from build123d import *

# Parameters (mm, degrees)
SKETCH1_R            = 1
BOSS_EXTRUDE1_DEPTH  = 6
SKETCH2_R            = 2.6
CUT_EXTRUDE1_DEPTH   = 6
SKETCH3_W            = 7.6
SKETCH3_H            = 13
BOSS_EXTRUDE2_DEPTH  = 6
BOSS_EXTRUDE5_START  = -5
SKETCH6_W            = 3
SKETCH6_H            = 2
BOSS_EXTRUDE5_DEPTH  = 13
BOSS_EXTRUDE6_START  = -6
SKETCH10_R           = 4
SKETCH10_R_2         = 2.6
BOSS_EXTRUDE6_DEPTH  = 1.5
BOSS_EXTRUDE7_START  = -6
SKETCH12_R           = 2.6
SKETCH12_R_2         = 2.4
BOSS_EXTRUDE7_DEPTH  = 2
CUT_EXTRUDE2_DEPTH   = 7
SKETCH14_W           = 3
SKETCH14_H           = 6
CUT_EXTRUDE3_DEPTH   = 2
SKETCH15_W           = 0.2
SKETCH15_H           = 13
CUT_EXTRUDE5_DEPTH   = 7.5
SKETCH16_W           = 3
SKETCH16_H           = 3
CUT_EXTRUDE6_DEPTH   = 3
SKETCH17_W           = 2.8
SKETCH17_H           = 2.8
BOSS_EXTRUDE9_DEPTH  = 3
BOSS_EXTRUDE10_START = 24.4
SKETCH17_2_W         = 2.8
SKETCH17_2_H         = 2.8
BOSS_EXTRUDE10_DEPTH = 3
SKETCH18_W           = 5.7
SKETCH18_H           = 13
SKETCH18_W_2         = 13.3
CUT_EXTRUDE7_DEPTH   = 9
SKETCH19_W           = 3
SKETCH19_H           = 3
CUT_EXTRUDE8_DEPTH   = 3
CUT_EXTRUDE10_START  = -24
SKETCH19_3_W         = 3
SKETCH19_3_H         = 3
CUT_EXTRUDE10_DEPTH  = 3


with BuildPart() as part:
    # Sketch1 → Boss-Extrude1 (new body)
    with BuildSketch(Plane.XY):
        with BuildLine():
            ThreePointArc((3.75, -5), (4.47902769, -4.358991965), (5.1, -3.61282438))
            Line((5.1, -3.61282438), (5.1, 3.61282438))
            ThreePointArc((5.1, 3.61282438), (0, 6.25), (-5.1, 3.61282438))
            Line((-5.1, 3.61282438), (-5.1, -3.61282438))
            ThreePointArc((-5.1, -3.61282438), (-4.47902769, -4.358991965), (-3.75, -5))
            Line((-3.75, -5), (-14.7, -5))
            Line((-14.7, -5), (-14.7, 8))
            Line((-14.7, 8), (14.7, 8))
            Line((14.7, 8), (14.7, -5))
            Line((14.7, -5), (3.75, -5))
        make_face()
        with Locations((11.5, 0)):
            Circle(SKETCH1_R, mode=Mode.SUBTRACT)
        with Locations((-11.5, 0)):
            Circle(SKETCH1_R, mode=Mode.SUBTRACT)
    extrude(amount=BOSS_EXTRUDE1_DEPTH)

    # Sketch2 → Cut-Extrude1 (cut)
    with BuildSketch(Plane.XY):
        with Locations((-11.5, 0)):
            Circle(SKETCH2_R)
        with Locations((11.5, 0)):
            Circle(SKETCH2_R)
    extrude(amount=CUT_EXTRUDE1_DEPTH, mode=Mode.SUBTRACT)

    # Sketch3 → Boss-Extrude2 (add)
    with BuildSketch(Plane.XY):
        with Locations((-18.5, 1.5)):
            Rectangle(SKETCH3_W, SKETCH3_H)
    extrude(amount=BOSS_EXTRUDE2_DEPTH)

    # Sketch6 → Boss-Extrude5 (add)
    with BuildSketch(Plane(origin=(0, 0, 0), x_dir=(1, 0, 0), z_dir=(0, 1, 0)).offset(BOSS_EXTRUDE5_START)):
        with Locations((-23.8, -3)):
            Rectangle(SKETCH6_W, SKETCH6_H)
        with Locations((16.2, -3)):
            Rectangle(SKETCH6_W, SKETCH6_H)
    extrude(amount=BOSS_EXTRUDE5_DEPTH)

    # Sketch10 → Boss-Extrude6 (add)
    with BuildSketch(Plane.XY.offset(6).offset(BOSS_EXTRUDE6_START)):
        with Locations((-11.5, 0)):
            Circle(SKETCH10_R)
        with Locations((-11.5, 0)):
            Circle(SKETCH10_R_2, mode=Mode.SUBTRACT)
        with BuildLine():
            Line((14.7, 2.4), (14.7, -2.4))
            ThreePointArc((14.7, -2.4), (7.5, 0), (14.7, 2.4))
        make_face()
        with Locations((11.5, 0)):
            Circle(SKETCH10_R_2, mode=Mode.SUBTRACT)
    extrude(amount=-BOSS_EXTRUDE6_DEPTH)

    # Sketch12 → Boss-Extrude7 (add)
    with BuildSketch(Plane(origin=(0, 0, 0), x_dir=(-1, 0, 0), z_dir=(0, 0, -1)).offset(BOSS_EXTRUDE7_START)):
        with Locations((11.5, 0)):
            Circle(SKETCH12_R)
        with Locations((11.5, 0)):
            Circle(SKETCH12_R_2, mode=Mode.SUBTRACT)
        with Locations((-11.5, 0)):
            Circle(SKETCH12_R)
        with Locations((-11.5, 0)):
            Circle(SKETCH12_R_2, mode=Mode.SUBTRACT)
    extrude(amount=BOSS_EXTRUDE7_DEPTH)

    # Sketch13 → Cut-Extrude2 (cut)
    with BuildSketch(Plane.XZ.offset(5)):
        Polygon((-22.3, 0), (-16.3, 0), (-16.3, 2), (-17.8, 2), (-17.8, 6), (-20.8, 6), (-20.8, 2), (-22.3, 2), align=None)
    extrude(amount=-CUT_EXTRUDE2_DEPTH, mode=Mode.SUBTRACT)

    # Sketch14 → Cut-Extrude3 (cut)
    with BuildSketch(Plane(origin=(0, 0, 0), x_dir=(-1, 0, 0), z_dir=(0, 0, -1))):
        with Locations((19.3, 5)):
            Rectangle(SKETCH14_W, SKETCH14_H)
    extrude(amount=-CUT_EXTRUDE3_DEPTH, mode=Mode.SUBTRACT)

    # Sketch15 → Cut-Extrude5 (cut, symmetric)
    with BuildSketch(Plane.XY):
        with Locations((-12.1, 1.5)):
            Rectangle(SKETCH15_W, SKETCH15_H)
        with Locations((12.1, 1.5)):
            Rectangle(SKETCH15_W, SKETCH15_H)
    extrude(amount=CUT_EXTRUDE5_DEPTH, both=True, mode=Mode.SUBTRACT)

    # Sketch16 → Cut-Extrude6 (cut)
    with BuildSketch(Plane(origin=(12, 0, 0), x_dir=(0, 0, -1), z_dir=(1, 0, 0))):
        with Locations((-3, 5.173669459)):
            Rectangle(SKETCH16_W, SKETCH16_H)
    cut_extrude6 = extrude(amount=-CUT_EXTRUDE6_DEPTH, mode=Mode.SUBTRACT)

    # Mirror1: Cut-Extrude6 across plane
    add(cut_extrude6.mirror(Plane(origin=(0, 0, 0), x_dir=(0, 0, 1), z_dir=(1, 0, 0))), mode=Mode.SUBTRACT)

    # Sketch17 → Boss-Extrude9 (add)
    with BuildSketch(Plane(origin=(-12.2, 0, 0), x_dir=(0, 0, -1), z_dir=(1, 0, 0))):
        with Locations((-3, 5.173669459)):
            Rectangle(SKETCH17_W, SKETCH17_H)
    extrude(amount=BOSS_EXTRUDE9_DEPTH)

    # Sketch17<2> → Boss-Extrude10 (add)
    with BuildSketch(Plane(origin=(-12.2, 0, 0), x_dir=(0, 0, -1), z_dir=(1, 0, 0)).offset(BOSS_EXTRUDE10_START)):
        with Locations((-3, 5.173669459)):
            Rectangle(SKETCH17_2_W, SKETCH17_2_H)
    extrude(amount=-BOSS_EXTRUDE10_DEPTH)

    # Sketch18 → Cut-Extrude7 (cut, symmetric)
    with BuildSketch(Plane.XY):
        with Locations((14.85, 1.5)):
            Rectangle(SKETCH18_W, SKETCH18_H)
        with Locations((-18.65, 1.5)):
            Rectangle(SKETCH18_W_2, SKETCH18_H)
    extrude(amount=CUT_EXTRUDE7_DEPTH, both=True, mode=Mode.SUBTRACT)

    # Sketch19 → Cut-Extrude8 (cut)
    with BuildSketch(Plane(origin=(12, 0, 0), x_dir=(0, 0, -1), z_dir=(1, 0, 0))):
        with Locations((-3, 5.173669459)):
            Rectangle(SKETCH19_W, SKETCH19_H)
    extrude(amount=-CUT_EXTRUDE8_DEPTH, mode=Mode.SUBTRACT)

    # Sketch19<3> → Cut-Extrude10 (cut)
    with BuildSketch(Plane(origin=(12, 0, 0), x_dir=(0, 0, -1), z_dir=(1, 0, 0)).offset(CUT_EXTRUDE10_START)):
        with Locations((-3, 5.173669459)):
            Rectangle(SKETCH19_3_W, SKETCH19_3_H)
    extrude(amount=CUT_EXTRUDE10_DEPTH, mode=Mode.SUBTRACT)


solid = part.part
Can you work these out from the model? Positions are in its coordinate system, mm. A direction names the side the tool comes from. Coordinates: 2 decimals unless noted, no trailing zeros. Loops run counter-clockwise (first coordinate to the right, second up) from the corner with the lowest first, then second, coordinate; pieces in that order, holes last. Notation, with made-up numbers: (81, 4) - (122, 4) arc R19 cw to (122, 8) - close; hole circle Ø2 at (66, -0.75). An arc over 180 degrees is marked (long way). Answer as a JSON object with one key per item and string values. Group by question number.
Item 1: If we section it at B-B (y = 4.25): List the corners of the cut face in (x, z) for me.
Item 2: If we mould it in two halves opening along X, with no side actions, what happens to faces 1 (the face through (-12, -4, 3)), 2 (the face through (8.9, 0.1, 1.3)), 3 (the face through (-11, 5, 4.5)), 4 (the face through (4.47, -4.37, 2.96))? For each: released by +X, released by -X, zero draft, split by the parting line, or undercut.
Item 3: If I drill on L1, parallel to Y at x = 11.5, z = 4.45; L2, parallel to Y at x = 11.5, z = 5.5; L3, parallel to Y at x = -11.5, z = 1.25, over which ranges is the centre line in solid material (lowest first)? Write a range as from..to.
Item 4: If we section it at D-D (y = 0): List the corners of the cut face in (x, z) for me.
Item 5: On a 3-axis mill with a long thin cutter (end or side, diameter ignored), from which of +Z, -Z, +X, -X, +Y, -Y can I reach the whole of each face in a straight line? I mean faces 5 (the face through (-12, 5, 1)), 6 (the face through (11, 5, 4.5)), 7 (the face through (-9, 5, 3)). Say none if no direction works.
Item 6: If we section it at C-C (z = 5.5): List the corners of the cut face in (x, y) for me, plus the area to 3 significant figures.
Item 7: For pin 1 (4 mm diameter, centred on x = -3.5, y = 0.5, fed in from -Z); pin 2 (1 mm diameter, centred on y = -1.5, z = 5, fed in from +X); pin 3 (3 mm diameter, centred on x = -1, z = 0, fed in from -Y), each with a flat end and sliding along its axis, tell me the tip position at first contact or that it passes through.
Item 8: If we section it at A-A (x = 11.5): List the corners of the cut face in (y, z) for me, plus the area to 3 significant figures.
Returned:
{
 "1": {"outline": "(-12, 0) - (-4.58, 0) - (-4.58, 6) - (-12, 6) - (-12, 4.5) - (-9, 4.5) - (-9, 1.5) - (-12, 1.5) - close; (4.58, 0) - (12, 0) - (12, 1.5) - (9, 1.5) - (9, 4.5) - (12, 4.5) - (12, 6) - (4.58, 6) - close"},
 "2": {"face 1": "released by -X", "face 2": "undercut", "face 3": "zero draft", "face 4": "undercut"},
 "3": {"L1": "y = -5..-2.4, 2.4..3.67, 6.67..8", "L2": "y = -5..-2.4, 2.4..8", "L3": "y = -5..-2.6, 2.6..8"},
 "4": {"outline": "(-9.1, 4) - (-8.9, 4) - (-8.9, -1.5) - (-7.5, -1.5) - (-7.5, 0) - (-5.1, 0) - (-5.1, 6) - (-9.1, 6) - close; (5.1, 0) - (7.5, 0) - (7.5, -1.5) - (8.9, -1.5) - (8.9, 4) - (9.1, 4) - (9.1, 6) - (5.1, 6) - close"},
 "5": {"face 5": "+Z, -Z, -X, +Y, -Y", "face 6": "+X", "face 7": "-X"},
 "6": {"outline": "(-12, -5) - (-3.75, -5) arc R6.25 cw to (-5.1, -3.61) - (-5.1, 3.61) arc R6.25 cw to (5.1, 3.61) - (5.1, -3.61) arc R6.25 cw to (3.75, -5) - (12, -5) - (12, -2.35) arc R2.4 cw (long way) to (12, 2.35) - (12, 8) - (-12, 8) - (-12, 2.35) arc R2.4 cw (long way) to (-12, -2.35) - close", "area": "184 mm²"},
 "7": {"pin 1": "stops at z = 0", "pin 2": "stops at x = 10.17", "pin 3": "stops at y = 5.73"},
 "8": {"outline": "(-5, 0) - (-4, 0) - (-4, -1.5) - (-2.6, -1.5) - (-2.6, 4) - (-2.4, 4) - (-2.4, 6) - (-5, 6) - close; (2.4, 4) - (2.6, 4) - (2.6, -1.5) - (4, -1.5) - (4, 0) - (8, 0) - (8, 6) - (2.4, 6) - close; hole (3.67, 1.5) - (6.67, 1.5) - (6.67, 4.5) - (3.67, 4.5) - close", "area": "42.8 mm²"}
}
